Geometry: final body of the model. Coordinates: model frame, mm. Face numbers are marked on the shaded views. A direction names the side the tool comes from. Round coordinates to 2 decimals unless told otherwise and drop trailing zeros. Write each loop counter-clockwise with the first axis right and the second up, starting at its lowest first coordinate (ties: lowest second). Pieces come first, ordered by that corner, then holes. Notation, with made-up numbers: (77, 2) -> (134, 2) arc R20 ccw to (134, 14) -> close; hole circle Ø7 at (45.5, 38). An arc over 180 degrees is marked (long way). Use one line per item in the form item = value. Start each with the question number.
1. Cut plane A-A, the plane x = 2.25. Return the cut outline in (y, z), plus the area to 3 significant figures.
2. Pin query (flat end, axial travel): pin 1 Ø2 at (x, y) = (5, 6.5) entering from -Z; pin 2 Ø1.6 at (x, z) = (-3.5, -4.5) entering from +Y. Return the tip coordinate at first contact, or that it passes through.
3. Reachability of the marked faces 5 and 6 from +Z, -Z, +X, -X, +Y, -Y: full face, straight path, thin tool, end or side. Return the list, or none.
4. Cut plane C-C, the plane y = 5.5. Return the cut outline in (x, z).
5. Cut plane B-B, the plane z = 4.25. Return the cut outline in (x, y), plus the area to 3 significant figures.
6. Draft query along X for the marked faces 1, 2, 3 and 4. Return one class per face: pulls with the +X half, pulls with the -X half, needs draft (parallel to the pull), parting line crosses it, or undercut.
7. Line query: L1, parallel to Y at x = -1, z = -4.5; L2, parallel to Z at x = 6.5, y = 7.75; L3, parallel to Z at x = -5.25, y = 6.75. Output: solid intervals per line, ascending.
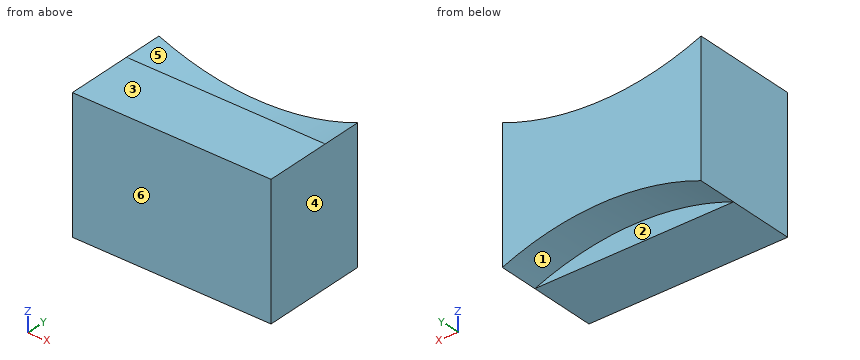
```python
from build123d import *

# Parameters (mm, degrees)
CROQUIS1_W              = 15
CROQUIS1_H              = 10
SALIENTE_EXTRUIR1_DEPTH = 8
CORTAR_EXTRUIR1_DEPTH   = 3


with BuildPart() as part:
    # Croquis1 → Saliente-Extruir1 (new body)
    with BuildSketch(Plane(origin=(0, 0, 0), x_dir=(1, 0, 0), z_dir=(0, 1, 0))):
        Rectangle(CROQUIS1_W, CROQUIS1_H)
    extrude(amount=SALIENTE_EXTRUIR1_DEPTH)

    # Croquis2 → Cortar-Extruir1 (cut)
    with BuildSketch(Plane(origin=(0, 8, 0), x_dir=(-1, 0, 0), z_dir=(0, 1, 0))):
        with BuildLine():
            ThreePointArc((7.5, -5), (0, -3.540496218), (-7.5, -5))
            Line((-7.5, -5), (7.5, -5))
        make_face()
        with BuildLine():
            ThreePointArc((7.5, 5), (0, 3.540496218), (-7.5, 5))
            Line((-7.5, 5), (7.5, 5))
        make_face()
    extrude(amount=-CORTAR_EXTRUIR1_DEPTH, mode=Mode.SUBTRACT)


solid = part.part
```
Outcome:
q1.outline = (0, -5) -> (5, -5) -> (5, -3.67) -> (8, -3.67) -> (8, 3.67) -> (5, 3.67) -> (5, 5) -> (0, 5) -> close
q1.area = 72.0 mm^2
q2.pin_1 = -4.46
q2.pin_2 = 8
q3.face_5 = +Z, +Y
q3.face_6 = +Z, -Z, +X, -X, -Y
q4.outline = (-7.5, -5) arc R20 cw to (7.5, -5) -> (7.5, 5) arc R20 cw to (-7.5, 5) -> close
q5.outline = (-7.5, 0) -> (7.5, 0) -> (7.5, 8) -> (5.28, 8) -> (5.28, 5) -> (-5.28, 5) -> (-5.28, 8) -> (-7.5, 8) -> close
q5.area = 88.3 mm^2
q6.face_1 = undercut
q6.face_2 = undercut
q6.face_3 = needs draft
q6.face_4 = pulls with the +X half
q7.L1 = 0 to 5
q7.L2 = -4.63 to 4.63
q7.L3 = -4.24 to 4.24
